Input: part model. Units: mm. Frame: model coordinates. A direction names the side the tool comes from. Coordinates: 2 decimals unless noted, no trailing zeros. One line per question, with ' | ' between items. Start each with the question number.
1) First-contact query: P1, Ø5, axis at x = 10, y = 12.5, coming from the +Z side; P2, Ø1, axis at y = 9, z = 13, coming from the +X side; P3, Ø3, axis at x = 12.7, z = -7.5, coming from the -Y side; P4, Ø5, axis at y = 8.5, z = -6.5, coming from the +X side. Flat tips, straight axial feed; report the tip coordinate or a pass-through.
2) Draft query along X for faces 1 (the cylindrical face through (23.97, 1.5, 16.82)), 2 (the cylindrical face through (1.504, 14.814, -7.093)), 3 (the cylindrical face through (12.51, 14.205, -2.504)), 4 (the conical face through (14.128, 21.808, -5.26)). Return one class per face: released by +X, released by -X, zero draft, split by the parting line, or undercut.
3) Reachability of faces 5 (the cylindrical face through (12.8, 0.7, 0.3)), 6 (the flat face through (15, 15, 5)) from +Z, -Z, +X, -X, +Y, -Y: full face, straight path, thin tool, end or side. Return the list, or none.
4) Line query: line 1 (X direction, y = 24.2, z = -7.5); line 2 (Z direction, x = 12.7, y = 7.75); line 3 (Y direction, x = 10, z = 14). Output: solid intervals per line, ascending.
```python
from build123d import *

# Parameters (mm, degrees)
F0_W     = 25.4
F0_H     = 25.4
F1_DEPTH = 5
F3_DEPTH = 25.4
F5_DEPTH = 25.4
F7_D     = 5
F9_D     = 10
F9_DEPTH = 20.4
F9_TIP   = 3.0043030951
F10_R    = 4.99999


# Not quite as in the source:
# - a fillet or chamfer is up to 0.001 mm smaller than in the source, because OpenCascade refuses the exact size


with BuildPart() as f1:
    # F0 (on Top) → F1 (new body)
    with BuildSketch(Plane.XY):
        with Locations((12.7, 12.7)):
            Rectangle(F0_W, F0_H)
    extrude(amount=F1_DEPTH)

    # F2 (on face) → F3 (join)
    with BuildSketch(Plane.XY.offset(5)):
        Polygon((5, 25.4), (0, 25.4), (0, 0), (25.4, 0), (25.4, 5), (5, 5), align=None)
    extrude(amount=F3_DEPTH)

    # F4 (on face) → F5 (join, through all)
    with BuildSketch(Plane.YZ.offset(25.4)):
        Polygon((25.4, -15), (25.4, 0), (0, 0), align=None)
    extrude(amount=-F5_DEPTH)

    # F7 (through all)
    with Locations(Plane.XZ):
        with Locations((12.7, -7.5)):
            Hole(F7_D / 2)

    # F9
    with Locations(Plane.XZ):
        with Locations((12.7, -7.5)):
            Hole(F9_D / 2, depth=F9_DEPTH)
            with Locations((0, 0, -(F9_DEPTH + F9_TIP / 2))):  # 118° drill point
                Cone(0, F9_D / 2, F9_TIP, mode=Mode.SUBTRACT)

    # F10 (radius 5 in the source; OpenCascade refuses exactly that, so slightly less here)
    f10_edges = [f1.edges().sort_by_distance(p)[0] for p in [
        (0, 0, 15.2),
        (0, 12.7, -7.5),
        (12.7, 0, 0),
        (25.4, 12.7, -7.5),
        (25.4, 0, 15.2),
        (12.7, 0, 30.4),
        (0, 12.7, 30.4),
    ]]
    fillet(f10_edges, radius=F10_R)


solid = f1.part
```
Answer key:
1) P1: z = 5 | P2: x = 5 | P3: through | P4: x = 23.68
2) face 1: released by +X | face 2: released by -X | face 3: undercut | face 4: undercut
3) face 5: -Z, +X, -X, -Y | face 6: +Z, +X, +Y
4) line 1: 0 to 10.2, 15.2 to 25.4 | line 2: -2.5 to 5 | line 3: 0 to 5
